Source: three-view drawing plus pictorial views. Frame: mm from the lowest corner of the part. A direction names the side the tool comes from. Coordinates: 2 decimals unless noted, no trailing zeros. Write each loop counter-clockwise with the first axis right and the second up, starting at its lowest first coordinate (ties: lowest second). Pieces come first, ordered by that corner, then holes. Notation, with made-up numbers: (89, 53.5) - (127, 53.5) arc R21 cw to (127, 60.5) - close; hole circle Ø6 at (-35.5, -14). An arc over 180 degrees is marked (long way). Put each result on its own line as item: value. Start each with the question number.
1. Cut plane D-D, the plane x = 14.5. Return loops of the section in (y, z), and give its area (3 significant figures).
2. Cut plane B-B, the plane z = 23. Return loops of the section in (x, y).
3. Pin query (flat end, axial travel): pin 1 (3 mm diameter, centred on x = 13.5, z = 9.5, fed in from -Y); pin 2 (4 mm diameter, centred on y = 7, z = 2, fed in from -X); pin 3 (5.5 mm diameter, centred on y = 4.5, z = 2, fed in from +X). Return the tip coordinate at first contact, or that it passes through.
4. Cut plane A-A, the plane y = 20. Return loops of the section in (x, z) (3 decimals).
5. Access query for the marked faces 4, 5 and 6. Directions: +Z, -Z, +X, -X, +Y, -Y. A direction counts if a zero-diameter tool reaches every point of the face in a straight line with its end or side. Return the directions, or none.
6. Cut plane C-C, the plane x = 8.25. Return loops of the section in (y, z) (3 decimals).
7. Pull-direction query (Y, two-part tool) for the marked faces 1, 2 and 3; classes: released by +Y, released by -Y, zero draft, split by the parting line, or undercut.
8. Line query: line 1 (Y direction, x = 8.25, z = 1.2) (3 decimals); line 2 (Y direction, x = 8.25, z = 2.9) (3 decimals); line 3 (Z direction, x = 4.75, y = 47.5). Output: solid intervals per line, ascending.
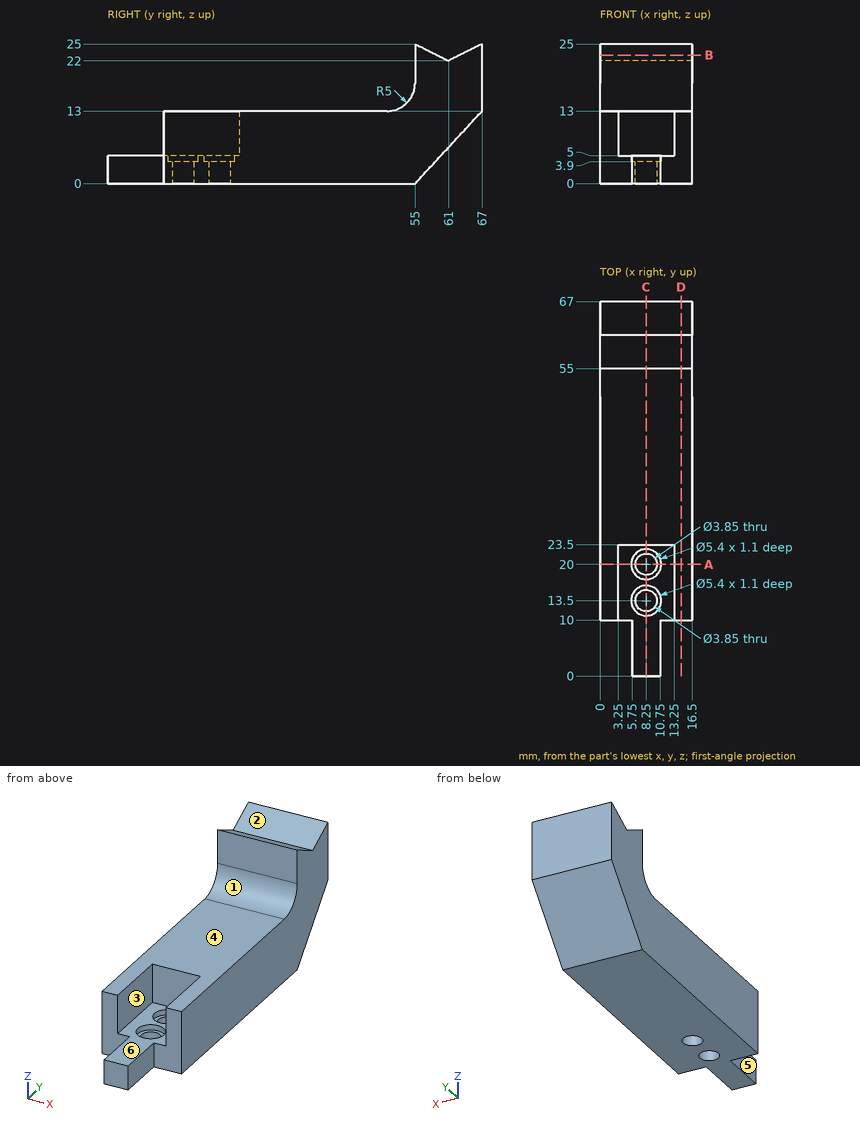
Report:
1. outline: (10, 0) - (55, 0) - (67, 13) - (67, 25) - (61, 22) - (55, 25) - (55, 18) arc R5 cw to (50, 13) - (10, 13) - close
1. area: 794 mm^2
2. outline: (0, 55) - (16.5, 55) - (16.5, 59) - (0, 59) - close; (0, 63) - (16.5, 63) - (16.5, 67) - (0, 67) - close
3. pin 1: stops at y = 10
3. pin 2: stops at x = 5.75
3. pin 3: stops at x = 10.75
4. outline: (0, 0) - (6.325, 0) - (6.325, 3.9) - (5.55, 3.9) - (5.55, 5) - (3.25, 5) - (3.25, 13) - (0, 13) - close; (10.175, 0) - (16.5, 0) - (16.5, 13) - (13.25, 13) - (13.25, 5) - (10.95, 5) - (10.95, 3.9) - (10.175, 3.9) - close
5. face 4: +Z, +X, -X, -Y
5. face 5: +Z, -Z, -X, -Y
5. face 6: +Z, -Y
6. outline: (0, 0) - (11.575, 0) - (11.575, 3.9) - (10.8, 3.9) - (10.8, 5) - (0, 5) - close; (15.425, 0) - (18.075, 0) - (18.075, 3.9) - (17.3, 3.9) - (17.3, 5) - (16.2, 5) - (16.2, 3.9) - (15.425, 3.9) - close; (21.925, 0) - (55, 0) - (67, 13) - (67, 25) - (61, 22) - (55, 25) - (55, 18) arc R5 cw to (50, 13) - (23.5, 13) - (23.5, 5) - (22.7, 5) - (22.7, 3.9) - (21.925, 3.9) - close
7. face 1: released by -Y
7. face 2: undercut
7. face 3: zero draft
8. line 1: y = 0 to 11.575, 15.425 to 18.075, 21.925 to 56.108
8. line 2: y = 0 to 11.575, 15.425 to 18.075, 21.925 to 57.677
8. line 3: z = 0 to 13
